Geometry: final body of the model. Coordinates: model frame, mm. Face numbers are marked on the shaded views. A direction names the side the tool comes from. Round coordinates to 2 decimals unless told otherwise and drop trailing zeros. Loops run counter-clockwise (first coordinate to the right, second up) from the corner with the lowest first, then second, coordinate; pieces in that order, holes last. Notation, with made-up numbers: (43.5, -9) - (59.5, -9) arc R29 cw to (59.5, 21) - close; hole circle Ø1 at (14.25, 35.5). An arc over 180 degrees is marked (long way). Answer as a JSON object with one key per item and string values. Group by question number.
Item 1: Reachability of the marked faces 5, 6 and 7 from +Z, -Z, +X, -X, +Y, -Y: full face, straight path, thin tool, end or side. Return the list, or none.
Item 2: First-contact query: pin 1 (5 mm diameter, centred on x = 42.5, y = -14.5, fed in from +Z); pin 2 (4 mm diameter, centred on x = 43, z = 22, fed in from -Y); pin 3 (4 mm diameter, centred on x = 42, z = 23.5, fed in from +Y). Flat tips, straight axial feed; report the tip coordinate or a pass-through.
Item 3: Line query: line 1 (Y direction, x = -11.5, z = 14.5); line 2 (Z direction, x = 8, y = -20) (3 decimals); line 3 (X direction, y = 2.5, z = 23.25). Output: solid intervals per line, ascending.
Item 4: Section D-D (z = 15.25). Return the cut outline in (x, y).
Item 5: Draft query along Y for the marked faces 1, 2, 3 and 4. Return one class per face: released by +Y, released by -Y, zero draft, split by the parting line, or undercut.
Item 6: Section A-A (z = 5). Return the cut outline in (x, y), plus the area to 3 significant figures.
Item 7: Section C-C (y = -20). Return the cut outline in (x, z) (3 decimals), plus the area to 3 significant figures.
Item 8: Section B-B (x = -20). Return the cut outline in (y, z) (3 decimals).
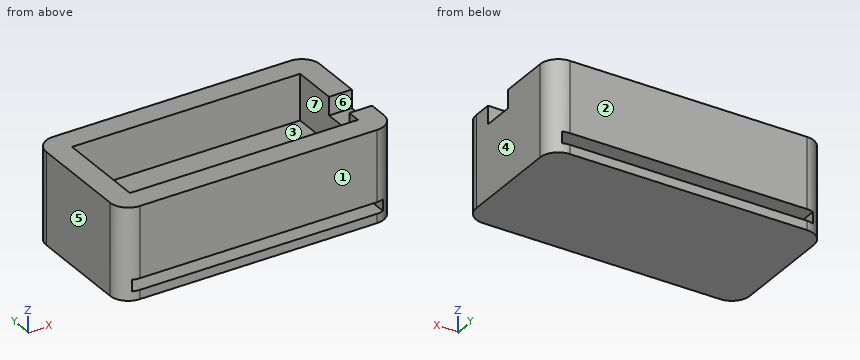
```python
from build123d import *

# Parameters (mm, degrees)
F0_W        = 76.2
F0_H        = 38.1
F1_DEPTH    = 25.4
F2_W        = 69.85
F2_H        = 3.175
F3_DEPTH    = 38.101
F4_W        = 63.5
F4_H        = 25.4
F5_DEPTH    = 12.7
F6_W        = 6.35
F6_H        = 8.89
F7_DEPTH    = 5.08
F8_T1_DEPTH = 50.8


# Not quite as in the source:
# - a fillet or chamfer that OpenCascade refuses, or shapes differently, is made with other operations: its cross-section is extruded or revolved along the edge and cut away or added


with BuildPart() as f1:
    # F0 (on Top) → F1 (new body)
    with BuildSketch(Plane.XY):
        with Locations((6.725884974, -8.772585205)):
            Rectangle(F0_W, F0_H)
    extrude(amount=F1_DEPTH)

    # F2 (on face) → F3 (cut, through all)
    with BuildSketch(Plane.XZ.offset(27.822585205)):
        with Locations((6.725884974, 4.1275)):
            Rectangle(F2_W, F2_H)
    extrude(amount=-F3_DEPTH, mode=Mode.SUBTRACT)

    # F4 (on face) → F5 (cut)
    with BuildSketch(Plane.XY.offset(25.4)):
        with Locations((6.725884974, -8.772585205)):
            Rectangle(F4_W, F4_H)
    extrude(amount=-F5_DEPTH, mode=Mode.SUBTRACT)

    # F6 (on face) → F7 (cut)
    with BuildSketch(Plane.XY.offset(25.4)):
        with Locations((41.650884974, -13.217585205)):
            Rectangle(F6_W, F6_H)
    extrude(amount=-F7_DEPTH, mode=Mode.SUBTRACT)

    # F8: fillet of radius 5.08 on 4 edges, made by hand

    # F8_s2 → F8_t1 (cut)
    with BuildSketch(Plane.XY.offset(-12.7)):
        with BuildLine():
            ThreePointArc((44.825884974, 5.197414795), (43.3379874224, 8.7895172434), (39.745884974, 10.277414795))
            Line((39.745884974, 10.277414795), (44.825884974, 10.277414795))
            Line((44.825884974, 10.277414795), (44.825884974, 5.197414795))
        make_face()
        with BuildLine():
            ThreePointArc((-26.294115026, 10.277414795), (-29.8862174744, 8.7895172434), (-31.374115026, 5.197414795))
            Line((-31.374115026, 5.197414795), (-31.374115026, 10.277414795))
            Line((-31.374115026, 10.277414795), (-26.294115026, 10.277414795))
        make_face()
        with BuildLine():
            ThreePointArc((44.825884974, -22.742585205), (43.3379874224, -26.3346876534), (39.745884974, -27.822585205))
            Line((39.745884974, -27.822585205), (44.825884974, -27.822585205))
            Line((44.825884974, -27.822585205), (44.825884974, -22.742585205))
        make_face()
        with BuildLine():
            ThreePointArc((-26.294115026, -27.822585205), (-29.8862174744, -26.3346876534), (-31.374115026, -22.742585205))
            Line((-31.374115026, -22.742585205), (-31.374115026, -27.822585205))
            Line((-31.374115026, -27.822585205), (-26.294115026, -27.822585205))
        make_face()
    extrude(amount=F8_T1_DEPTH, mode=Mode.SUBTRACT)


solid = f1.part
```
Values:
{
 "1": {"face 5": "+Z, -Z, -X, +Y, -Y", "face 6": "+Z, +X", "face 7": "+Z"},
 "2": {"pin 1": "stops at z = 20.32", "pin 2": "stops at y = -27.67", "pin 3": "stops at y = 10.27"},
 "3": {"line 1": "y = -27.82 to -21.47, 3.93 to 10.28", "line 2": "z = 0 to 2.54, 5.715 to 12.7", "line 3": "x = -31.37 to -25.02, 38.48 to 44.83"},
 "4": {"outline": "(-31.37, -22.74) arc R5.08 ccw to (-26.29, -27.82) - (39.75, -27.82) arc R5.08 ccw to (44.83, -22.74) - (44.83, 5.2) arc R5.08 ccw to (39.75, 10.28) - (-26.29, 10.28) arc R5.08 ccw to (-31.37, 5.2) - close; hole (-25.02, -21.47) - (38.48, -21.47) - (38.48, 3.93) - (-25.02, 3.93) - close"},
 "5": {"face 1": "released by -Y", "face 2": "released by +Y", "face 3": "undercut", "face 4": "zero draft"},
 "6": {"outline": "(-31.37, -22.74) arc R5.08 ccw to (-28.2, -27.45) - (-28.2, 9.91) arc R5.08 ccw to (-31.37, 5.2) - close; (41.65, -27.45) arc R5.08 ccw to (44.83, -22.74) - (44.83, 5.2) arc R5.08 ccw to (41.65, 9.91) - close", "area": "221 mm^2"},
 "7": {"outline": "(-31.374, 0) - (44.826, 0) - (44.826, 25.4) - (38.476, 25.4) - (38.476, 12.7) - (-25.024, 12.7) - (-25.024, 25.4) - (-31.374, 25.4) - close; hole (-28.199, 2.54) - (41.651, 2.54) - (41.651, 5.715) - (-28.199, 5.715) - close", "area": "907 mm^2"},
 "8": {"outline": "(-27.823, 0) - (10.277, 0) - (10.277, 2.54) - (-27.823, 2.54) - close; (-27.823, 5.715) - (10.277, 5.715) - (10.277, 25.4) - (3.927, 25.4) - (3.927, 12.7) - (-21.473, 12.7) - (-21.473, 25.4) - (-27.823, 25.4) - close"}
}
